Verification items for the finished model (mm, model axes). Face numbers are marked on the shaded views. A direction names the side the tool comes from. Round coordinates to 2 decimals unless told otherwise and drop trailing zeros. Write each loop counter-clockwise with the first axis right and the second up, starting at its lowest first coordinate (ties: lowest second). Pieces come first, ordered by that corner, then holes. Notation, with made-up numbers: M -34.75,30 L 19.25,30 A7 cw 19.25,43 Z; hole C -12.75,58.25 d5. An arc over 180 degrees is marked long. Write each question's results on one line, items separated by ' | '.
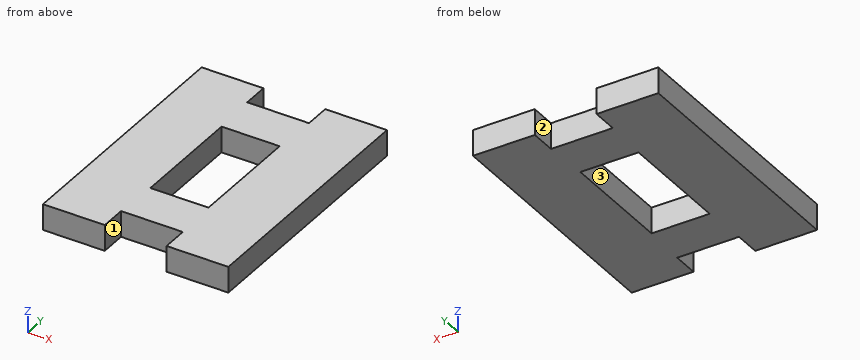
from build123d import *

# Parameters (mm, degrees)
SKETCH1_W           = 38.1
SKETCH1_H           = 52.07
BOSS_EXTRUDE1_DEPTH = 5.334
SKETCH2_W           = 11.938
SKETCH2_H           = 23.368
CUT_EXTRUDE1_DEPTH  = 54.818475018
SKETCH3_W           = 12.7
SKETCH3_H           = 5.334
CUT_EXTRUDE2_DEPTH  = 54.818475018


with BuildPart() as part:
    # Sketch1 → Boss-Extrude1 (new body)
    with BuildSketch(Plane.XY):
        with Locations((4.493611175, -22.065676399)):
            Rectangle(SKETCH1_W, SKETCH1_H)
    extrude(amount=BOSS_EXTRUDE1_DEPTH)

    # Sketch2 → Cut-Extrude1 (cut, through all)
    with BuildSketch(Plane.XY.offset(5.334)):
        with Locations((4.493611175, -22.065676399)):
            Rectangle(SKETCH2_W, SKETCH2_H)
    extrude(amount=-CUT_EXTRUDE1_DEPTH, mode=Mode.SUBTRACT)

    # Sketch3 → Cut-Extrude2 (cut, through all)
    with BuildSketch(Plane.XY.offset(5.334)):
        with Locations((4.493611175, 1.302323601)):
            Rectangle(SKETCH3_W, SKETCH3_H)
        with Locations((4.493611175, -45.433676399)):
            Rectangle(SKETCH3_W, SKETCH3_H)
    extrude(amount=-CUT_EXTRUDE2_DEPTH, mode=Mode.SUBTRACT)


solid = part.part
1) Access from +Z, -Z, +X, -X, +Y, -Y to the whole of each face (thin tool, end or side, straight path). Record for the marked faces 1, 2 and 3.
Calculated:
face 1: +Z, -Z, -Y | face 2: +Z, -Z, +Y | face 3: +Z, -Z
2) Sectioned sample at A-A, the plane y = 0.5. Record the cut outline in (x, z), and give its area (3 significant figures).
Calculated:
outline: M -14.56,0 L -1.86,0 L -1.86,5.33 L -14.56,5.33 Z; M 10.84,0 L 23.54,0 L 23.54,5.33 L 10.84,5.33 Z | area: 135 mm²
3) Sectioned sample at B-B, the plane x = 8. Record the cut outline in (y, z).
Calculated:
outline: M -42.77,0 L -33.75,0 L -33.75,5.33 L -42.77,5.33 Z; M -10.38,0 L -1.36,0 L -1.36,5.33 L -10.38,5.33 Z
4) Sectioned sample at C-C, the plane z = 1.05. Record the cut outline in (x, y).
Calculated:
outline: M -14.56,-48.1 L -1.86,-48.1 L -1.86,-42.77 L 10.84,-42.77 L 10.84,-48.1 L 23.54,-48.1 L 23.54,3.97 L 10.84,3.97 L 10.84,-1.36 L -1.86,-1.36 L -1.86,3.97 L -14.56,3.97 Z; hole M -1.48,-33.75 L 10.46,-33.75 L 10.46,-10.38 L -1.48,-10.38 Z
5) Material ranges on line 1 (X direction, y = -23, z = 2.9); line 2 (X direction, y = 0.5, z = 0.85); line 3 (Y direction, x = 4, z = 2), recorded low to high. Write a range as [from, to].
Calculated:
line 1: x = [-14.56, -1.48], [10.46, 23.54] | line 2: x = [-14.56, -1.86], [10.84, 23.54] | line 3: y = [-42.77, -33.75], [-10.38, -1.36]
6) Depth check by flat-ended pin: P1, Ø2.5, axis at x = 5, z = 2.5, coming from the -Y side; P2, Ø6, axis at x = -7.5, y = -7.5, coming from the -Z side; P3, Ø2.5, axis at x = 3.5, z = 2.5, coming from the +Y side. Enter the tip coordinate at first touch or a pass-through.
Calculated:
P1: stops at y = -42.77 | P2: stops at z = 0 | P3: stops at y = -1.36
